Check sheet for the modelled part. Datum: model origin and axes. Units: mm. Face numbers are marked on the shaded views. A direction names the side the tool comes from. Round coordinates to 2 decimals unless told otherwise and drop trailing zeros. Write each loop counter-clockwise with the first axis right and the second up, starting at its lowest first coordinate (ties: lowest second). Pieces come first, ordered by that corner, then holes.
Item 1: Section check C-C, the plane z = 0. Record the cut outline in (x, y).
Item 2: Material ranges on line 1 along X through (y, z) = (97.5, -289.5); line 2 along Y through (x, z) = (-365, 498); line 3 along Z through (x, y) = (-315.5, 78.5), recorded low to high.
Item 3: Depth check by flat-ended pin: pin 1 (8 mm diameter, centred on x = 231, z = -426, fed in from +Y); pin 2 (10 mm diameter, centred on y = 105.5, z = 416, fed in from +X); pin 3 (6 mm diameter, centred on x = -294, y = 74, fed in from +Z). Enter the tip coordinate at first touch or a pass-through.
Item 4: Section check B-B, the plane x = -300. Record the cut outline in (y, z).
Item 5: Section check D-D, the plane z = -203.5. Record the cut outline in (x, y).
Item 6: Section check A-A, the plane y = 54. Record the cut outline in (x, z), plus the area to 3 significant figures.
Item 7: Set-up check for the marked faces 1 and 2: record each of +Z, -Z, +X, -X, +Y, -Y from which the full face is reachable in a straight line by a thin tool's end or side.
from build123d import *

# Parameters (mm, degrees)
SKETCH2_W           = 1500
SKETCH2_H           = 1500
BOSS_EXTRUDE1_DEPTH = 10
SKETCH3_W           = 20
SKETCH3_H           = 1500
BOSS_EXTRUDE2_DEPTH = 110
SKETCH4_R           = 25
BOSS_EXTRUDE3_DEPTH = 110


with BuildPart() as part:
    # Sketch2 → Boss-Extrude1 (new body)
    with BuildSketch(Plane(origin=(0, 0, 0), x_dir=(1, 0, 0), z_dir=(0, 1, 0))):
        Rectangle(SKETCH2_W, SKETCH2_H)
    extrude(amount=BOSS_EXTRUDE1_DEPTH)

    # Sketch3 → Boss-Extrude2 (add)
    with BuildSketch(Plane(origin=(0, 10, 0), x_dir=(1, 0, 0), z_dir=(0, 1, 0))):
        with Locations((-610, 0)):
            Rectangle(SKETCH3_W, SKETCH3_H)
        with Locations((610, 0)):
            Rectangle(SKETCH3_W, SKETCH3_H)
    extrude(amount=BOSS_EXTRUDE2_DEPTH)

    # Sketch4 → Boss-Extrude3 (add)
    with BuildSketch(Plane(origin=(0, 10, 0), x_dir=(1, 0, 0), z_dir=(0, 1, 0))):
        with Locations((-300, 0)):
            Circle(SKETCH4_R)
    extrude(amount=BOSS_EXTRUDE3_DEPTH)


solid = part.part
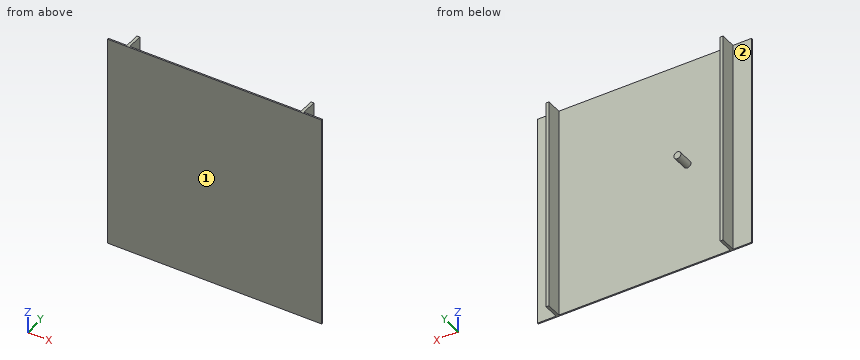
Values found:
1. outline: (-750, 0) - (750, 0) - (750, 10) - (620, 10) - (620, 120) - (600, 120) - (600, 10) - (-275, 10) - (-275, 120) - (-325, 120) - (-325, 10) - (-600, 10) - (-600, 120) - (-620, 120) - (-620, 10) - (-750, 10) - close
2. line 1: x = -620 to -600, 600 to 620
2. line 2: y = 0 to 10
2. line 3: z = -19.62 to 19.62
3. pin 1: stops at y = 10
3. pin 2: stops at x = 620
3. pin 3: stops at z = 24.82
4. outline: (0, -750) - (10, -750) - (10, -25) - (120, -25) - (120, 25) - (10, 25) - (10, 750) - (0, 750) - close
5. outline: (-750, 0) - (750, 0) - (750, 10) - (620, 10) - (620, 120) - (600, 120) - (600, 10) - (-600, 10) - (-600, 120) - (-620, 120) - (-620, 10) - (-750, 10) - close
6. outline: (-620, -750) - (-600, -750) - (-600, 750) - (-620, 750) - close; circle Ø50 at (-300, 0); (600, -750) - (620, -750) - (620, 750) - (600, 750) - close
6. area: 62,000 mm2
7. face 1: +Z, -Z, +X, -X, -Y
7. face 2: +Z, -Z, -X, +Y
